```python
from build123d import *

# Parameters (mm, degrees)
SWEEP1_PROFILE_R = 13.589
SWEEP2_PROFILE_R = 6.35
SHELL1_T         = -1.524


with BuildPart() as part:
    # Sweep1: sweep along a path in Sketch2
    with BuildLine(Plane.YZ) as sweep1_path:
        Line((-838.2, 89.789), (0, 89.789))
        ThreePointArc((0, 89.789), (89.789, 0), (0, -89.789))
        Line((0, -89.789), (-838.2, -89.789))
    # Sweep1 profile (on start of the path) → Sweep1 (sweep)
    with BuildSketch(Plane(origin=(0, -838.2, 89.789), x_dir=(0, 0, 1), z_dir=(0, 1, 0))):
        Circle(SWEEP1_PROFILE_R)
    sweep(path=sweep1_path.line)

    # Sweep2: sweep along a path in Sketch2<3>
    with BuildLine(Plane.YZ) as sweep2_path:
        Line((-685.8, 89.789), (-685.8, -89.789))
    # Sweep2 profile (on start of the path) → Sweep2 (sweep)
    with BuildSketch(Plane(origin=(0, -685.8, 89.789), x_dir=(-1, 0, 0), z_dir=(0, 0, -1))):
        Circle(SWEEP2_PROFILE_R)
    sweep(path=sweep2_path.line)

    # Shell1
    shell1_openings = [part.faces().sort_by_distance(p)[0] for p in [
        (0, -838.2, 89.789),
        (0, -838.2, -89.789),
    ]]
    offset(amount=SHELL1_T, openings=shell1_openings, kind=Kind.INTERSECTION)


solid = part.part
```
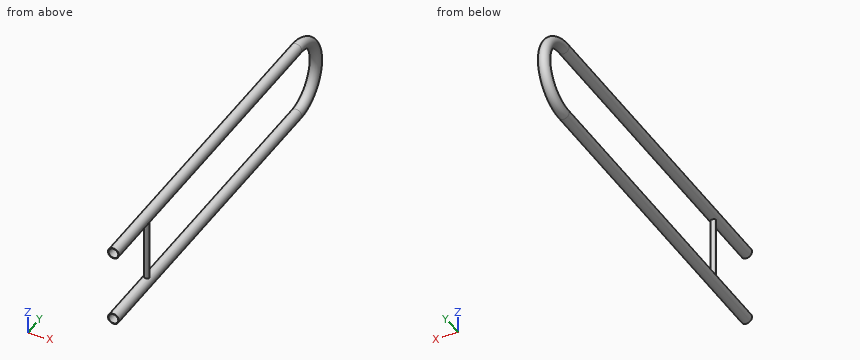
CAD build for the part. Positions are in the model's coordinates, mm. Round coordinates to 2 decimals unless told otherwise and drop trailing zeros. Loops run counter-clockwise (first coordinate to the right, second up) from the corner with the lowest first, then second, coordinate; pieces in that order, holes last. Notation, with made-up numbers: M -29.75,79 L -16.75,79 A32 ccw -16.75,113 Z; hole C 49,-24.5 d9. An arc over 180 degrees is marked long. Use a Markdown table: item, result. Add a question column.
(1) Flat gauge pins, fed straight in: pin 1 (10 mm diameter, centred on x = 6, z = 25, fed in from -Y); pin 2 (3 mm diameter, centred on x = -3, z = -66.5, fed in from +Y); pin 3 (4 mm diameter, centred on x = 1, z = -8, fed in from +Y). Where does each tip first touch, or does it go through?
(2) Drill centre lines: line 1 (Z direction, x = 0, y = -569); line 2 (Z direction, x = 1.25, y = -271); line 3 (X direction, y = -685.8, z = 8.5). Where is each one in solid material? Low to high.
(3) Cut at C-C (z = 58). State how many separate pieces and enclosed holes the cut face has, and give its area (3 significant figures).
(4) Cut at A-A (x = 0). Give the cut face in (y, z).
(5) Cut at B-B (y = -237.5). Give the cut face in (x, z) (3 decimals).
Geometry says:
| question | item | result |
|---|---|---|
| 1 | pin 1 | stops at y = -692.07 |
| 1 | pin 2 | stops at y = 80.02 |
| 1 | pin 3 | stops at y = 103.19 |
| 2 | line 1 | z = -103.38 to -101.85, -77.72 to -76.2, 76.2 to 77.72, 101.85 to 103.38 |
| 2 | line 2 | z = -103.32 to -101.79, -77.79 to -76.26, 76.26 to 77.79, 101.79 to 103.32 |
| 2 | line 3 | x = -6.35 to -4.83, 4.83 to 6.35 |
| 3 | separate pieces | 2 |
| 3 | enclosed holes | 2 |
| 3 | area | 218 mm² |
| 4 | outline | M -838.2,-103.38 L 0,-103.38 A103.38 ccw 0,103.38 L -838.2,103.38 L -838.2,101.85 L 0,101.85 A101.85 cw 0,-101.85 L -838.2,-101.85 Z; M -838.2,-77.72 L -690.63,-77.72 L -690.63,77.72 L -838.2,77.72 L -838.2,76.2 L -692.15,76.2 L -692.15,-76.2 L -838.2,-76.2 Z; M -680.97,-77.72 L 0,-77.72 A77.72 ccw 0,77.72 L -680.97,77.72 Z; hole M -679.45,-76.2 L 0,-76.2 A76.2 ccw 0,76.2 L -679.45,76.2 Z |
| 5 | outline | C 0,-89.789 d27.178; C 0,89.789 d27.178; hole C 0,-89.789 d24.13; hole C 0,89.789 d24.13 |
